Autodesk Inventor part; units mm, degrees
ref_plane "YZ Plane" through (0, 0, 0) normal (1, 0, 0) x (0, 1, 0)
ref_plane "XZ Plane" through (0, 0, 0) normal (0, 1, 0) x (-1, 0, 0)
ref_plane "XY Plane" through (0, 0, 0) normal (0, 0, 1) x (1, 0, 0)
sketch "Sketch1" plane through (0, 0, 0) normal (0, 0, 1) x (1, 0, 0)
  circle A0 centre (0, 0) radius 2.8166
extrude "Extrusion1" add sketch "Sketch1" along normal blind 14.2875
sketch "Sketch2" plane through (0, 0, 14.2875) normal (0, 0, 1) x (1, 0, 0)
  circle A0 centre (0, 0) radius 0.8892
extrude "Extrusion2" add sketch "Sketch2" along normal blind 1.5875
sketch "Sketch3" plane through (0, 0, 15.875) normal (0, 0, 1) x (1, 0, 0)
  circle A0 centre (0, 0) radius 3.1943
extrude "Extrusion3" add sketch "Sketch3" along normal blind 0.508
sketch "Sketch4" plane through (0, 0, 16.383) normal (0, 0, 1) x (1, 0, 0)
  point P0 (0, 0)
sketch "Sketch5" plane through (0, 0, 16.383) normal (0, 0, 1) x (1, 0, 0)
  circle A0 centre (0, 0) radius 3.1943
  circle A1 centre (2.0744, 0) radius 0.5486
  circle A2 centre (0, -2.0828) radius 0.5461
  circle A3 centre (-2.0828, 0) radius 0.5461
  circle A4 centre (0, 2.0828) radius 0.5461
extrude "Extrusion4" cut sketch "Sketch5" against normal blind 0.508 contours A1 | A2 | A3 | A4
sketch "Sketch6" plane through (0, 0, 16.383) normal (0, 0, 1) x (1, 0, 0)
  point P0 (0, 0)
properties part number "Cylinder"
The model under review builds one solid part; all positions refer to its coordinate system, in mm. A direction names the side the tool comes from. Round coordinates to 2 decimals unless told otherwise and drop trailing zeros. Write each loop counter-clockwise with the first axis right and the second up, starting at its lowest first coordinate (ties: lowest second). Pieces come first, ordered by that corner, then holes. Notation, with made-up numbers: (68, 39.5) - (125, 39.5) arc R29 ccw to (125, 63.5) - close; hole circle Ø9 at (-21.75, 72). An arc over 180 degrees is marked (long way). Use one line per item in the form item = value.
Q1. Tool access review of faces 5 (the flat face through (1, -1, 15.875)), 6 (the flat face through (0, 0, 16.383)), 7 (the cylindrical face through (-0.071, 2.624, 16.133)): name each direction out of +Z, -Z, +X, -X, +Y, -Y from which nothing blocks a thin tool from reaching the whole face with its end or side.
Answer key:
face_5 = none
face_6 = +Z, +X, -X, +Y, -Y
face_7 = +Z
Q2. Consider section A-A (y = 0). State the section outline as (x, z) points (1 decimal), and give its area (3 significant figures).
Answer key:
outline = (-3.2, 15.9) - (-2.6, 15.9) - (-2.6, 16.4) - (-3.2, 16.4) - close; (-2.8, 0) - (2.8, 0) - (2.8, 14.3) - (0.9, 14.3) - (0.9, 15.9) - (1.5, 15.9) - (1.5, 16.4) - (-1.5, 16.4) - (-1.5, 15.9) - (-0.9, 15.9) - (-0.9, 14.3) - (-2.8, 14.3) - close; (2.6, 15.9) - (3.2, 15.9) - (3.2, 16.4) - (2.6, 16.4) - close
area = 85.4 mm2
Q3. Insertion check: pin 1 Ø3 at (x, y) = (1.5, -2.5) entering from -Z; pin 2 Ø3 at (y, z) = (-2.5, 9) entering from +X; pin 3 Ø1.5 at (y, z) = (1, 6) entering from -X; pin 4 Ø1 at (y, z) = (1.5, 5) entering from -X. Each pin has a flat end and moves straight along its axis. Give the tip position at first contact, or say it passes through.
Answer key:
pin_1 = 0
pin_2 = 2.63
pin_3 = -2.81
pin_4 = -2.63
Q4. Consider section C-C (x = -1.25). State the section outline as (y, z) points (1 decimal).
Answer key:
outline = (-2.9, 15.9) - (2.9, 15.9) - (2.9, 16.4) - (-2.9, 16.4) - close; (-2.5, 0) - (2.5, 0) - (2.5, 14.3) - (-2.5, 14.3) - close
Q5. For line 1 (Y direction, x = 0, z = 16.1); line 2 (Z direction, x = 0.5, y = 1) (1 decimal); line 3 (Y direction, x = -1, z = 2), list the stretches that pass through material, from the lowest coordinate up. Write a range as [from, to].
Answer key:
line_1 = [-3.19, -2.63], [-1.54, 1.54], [2.63, 3.19]
line_2 = [0, 14.3], [15.9, 16.4]
line_3 = [-2.63, 2.63]
Q6. Consider section D-D (z = 11.75). State the section outline as (x, y) points, and give its area (3 significant figures).
Answer key:
outline = circle Ø5.63 at (0, 0)
area = 24.9 mm2
Q7. Draft analysis for pull direction Y (two halves, no side actions). For faces 1 (the cylindrical face through (-0.07, -1.54, 16.13)), 2 (the cylindrical face through (-2.08, -1.9, 7.04)), 3 (the cylindrical face through (-2.63, 0.02, 16.13)), 4 (the flat face through (0, 0, 0)), state which applies: +Y half, -Y half, draft (parallel to the pull), parting line (faces both ways), or undercut.
Answer key:
face_1 = undercut
face_2 = parting line
face_3 = undercut
face_4 = draft
